Job drawing, mm, ordinate dimensions from the low corner. One solid piece. A direction names the side the tool comes from. Give positions to 0.01 mm unless a question says otherwise; leave off trailing zeros. Write each loop counter-clockwise with the first axis right and the second up, starting at its lowest first coordinate (ties: lowest second). Pieces come first, ordered by that corner, then holes. Notation, with made-up numbers: (86, -6.5) - (117, -6.5) arc R4 cw to (117, -2.5) - close; hole circle Ø9 at (20, 34.25). An arc over 180 degrees is marked (long way). Answer as a JSON object with one key per item and string values.
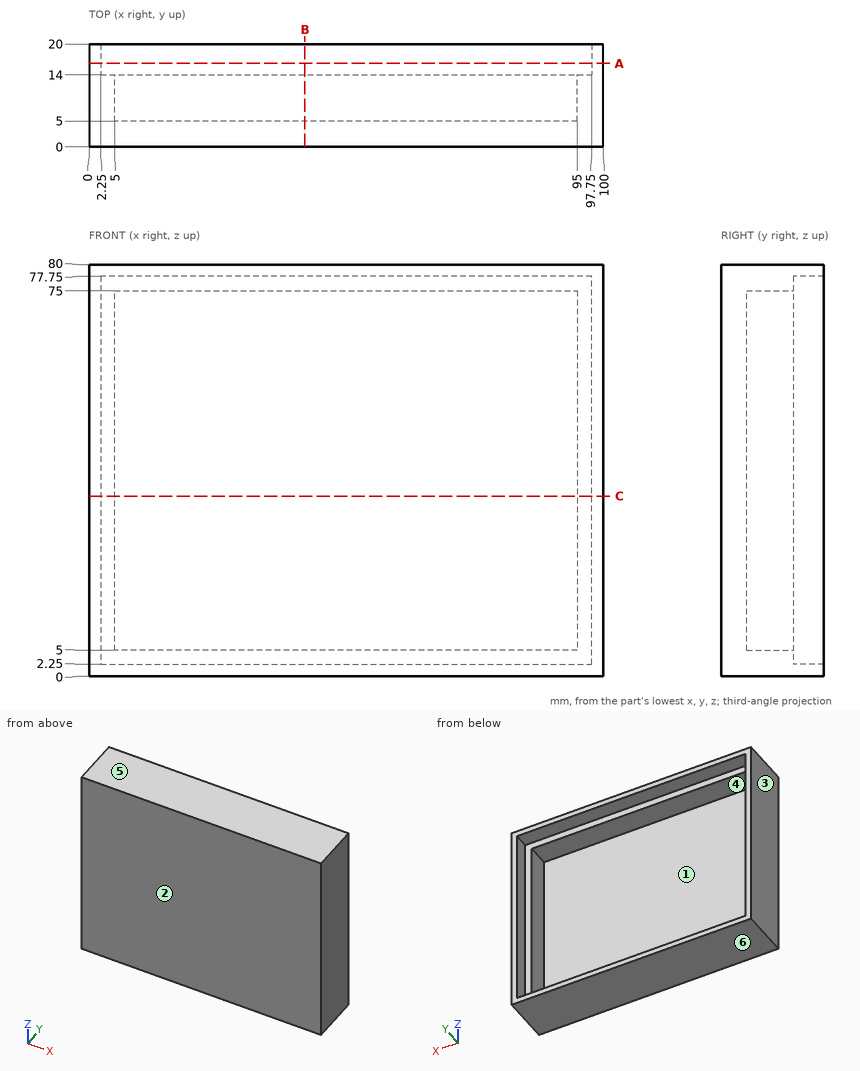
Item 1: Mould opens along Z. For the marked faces 3, 4, 5 and 6 say: +Z half, -Z half, draft (parallel to the pull), parting line (faces both ways), or undercut.
Entries:
{"face 3": "draft", "face 4": "undercut", "face 5": "+Z half", "face 6": "-Z half"}
Item 2: Cut at B-B (x = 42). Give the cut face in (y, z).
Entries:
{"outline": "(0, 0) - (20, 0) - (20, 2.25) - (14, 2.25) - (14, 5) - (5, 5) - (5, 75) - (14, 75) - (14, 77.75) - (20, 77.75) - (20, 80) - (0, 80) - close"}
Item 3: Cut at A-A (y = 16.25). Give the cut face in (x, z).
Entries:
{"outline": "(0, 0) - (100, 0) - (100, 80) - (0, 80) - close; hole (2.25, 2.25) - (97.75, 2.25) - (97.75, 77.75) - (2.25, 77.75) - close"}
Item 4: Probe line 1 (Z direction, x = 22, y = 5.5); line 2 (X direction, y = 11.25, z = 66.5); line 3 (Z direction, x = 53, y = 19). List the from-to ranges inside material, lowest first. Write a range as from..to.
Entries:
{"line 1": "0..5, 75..80", "line 2": "0..5, 95..100", "line 3": "0..2.25, 77.75..80"}
Item 5: Which spindle directions (+Z, -Z, +X, -X, +Y, -Y) get a long thin tool onto all of the face, cutting with end or side? Do the marked faces 1 and 2. Say none if no direction does.
Entries:
{"face 1": "+Y", "face 2": "+Z, -Z, +X, -X, -Y"}
Item 6: Cut at C-C (z = 35). Give the cut face in (x, y), and give its area (3 significant figures).
Entries:
{"outline": "(0, 0) - (100, 0) - (100, 20) - (97.75, 20) - (97.75, 14) - (95, 14) - (95, 5) - (5, 5) - (5, 14) - (2.25, 14) - (2.25, 20) - (0, 20) - close", "area": "617 mm2"}
Item 7: Flat gauge pins, fed straight in: P1, Ø6, axis at y = 8, z = 38, coming from the -X side; P2, Ø22.5, axis at x = 67, z = 25.5, coming from the +Y side; P3, Ø10, axis at x = 34.5, z = 8.5, coming from the +Y side. Where does each tip first touch, or does it go through?
Entries:
{"P1": "x = 0", "P2": "y = 5", "P3": "y = 14"}
